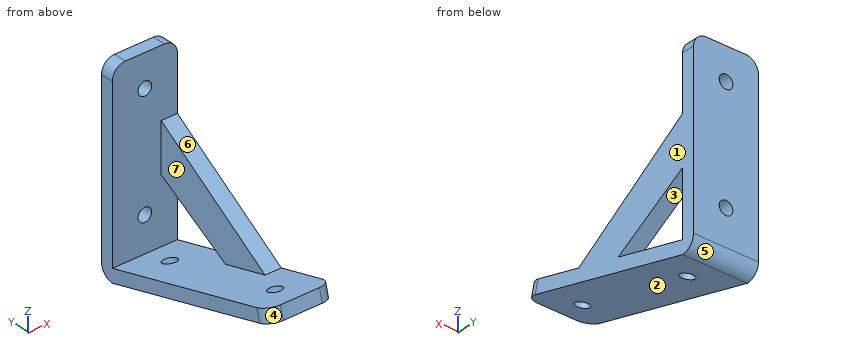
from build123d import *

# Parameters (mm, degrees)
SKETCH1_W           = 20
SKETCH1_H           = 60
BOSS_EXTRUDE1_DEPTH = 4
SKETCH6_W           = 20
SKETCH6_H           = 60
BOSS_EXTRUDE3_DEPTH = 4
FILLET6_R           = 4
SKETCH7_R           = 2.1
CUT_EXTRUDE3_DEPTH  = 4
SKETCH8_R           = 2.1
CUT_EXTRUDE4_DEPTH  = 4
FILLET7_R           = 4
FILLET8_R           = 4
FILLET9_R           = 4
FILLET10_R          = 4
BOSS_EXTRUDE5_DEPTH = 5


with BuildPart() as part:
    # Sketch1 → Boss-Extrude1 (new body)
    with BuildSketch(Plane(origin=(0, 0, 0), x_dir=(1, 0, 0), z_dir=(0, 1, 0))):
        Rectangle(SKETCH1_W, SKETCH1_H)
    extrude(amount=BOSS_EXTRUDE1_DEPTH)

    # Sketch6 → Boss-Extrude3 (add)
    with BuildSketch(Plane(origin=(0, -7.5, -27.990381057), x_dir=(-1, 0, 0), z_dir=(0, -0.25881904510251796, -0.9659258262890691))):
        with Locations((0, -22.235428647)):
            Rectangle(SKETCH6_W, SKETCH6_H)
    extrude(amount=-BOSS_EXTRUDE3_DEPTH)

    # Fillet6
    fillet6_edges = [part.edges().sort_by_distance(p)[0] for p in [
        (0, 4, -30),
    ]]
    fillet(fillet6_edges, radius=FILLET6_R - 0.0001)  # a hair under: the kernel refuses the full size

    # Sketch7 → Cut-Extrude3 (cut)
    with BuildSketch(Plane.XZ):
        with Locations(Location((0, 20, 0), (0, 0, 270))):
            Circle(SKETCH7_R)
        with Locations(Location((0, -15, 0), (0, 0, 270))):
            Circle(SKETCH7_R)
    extrude(amount=-CUT_EXTRUDE3_DEPTH, mode=Mode.SUBTRACT)

    # Sketch8 → Cut-Extrude4 (cut)
    with BuildSketch(Plane(origin=(0, -6.46472382, -24.126677752), x_dir=(1, 0, 0), z_dir=(0, 0.25881904510251796, 0.9659258262890691))):
        with Locations(Location((0, -2.771327032, 0), (0, 0, 270))):
            Circle(SKETCH8_R)
        with Locations(Location((0, -42.771327032, 0), (0, 0, 270))):
            Circle(SKETCH8_R)
    extrude(amount=-CUT_EXTRUDE4_DEPTH, mode=Mode.SUBTRACT)

    # Fillet7
    fillet7_edges = [part.edges().sort_by_distance(p)[0] for p in [
        (-10, -57.437911487, -12.539005641),
    ]]
    fillet(fillet7_edges, radius=FILLET7_R)

    # Fillet8
    fillet8_edges = [part.edges().sort_by_distance(p)[0] for p in [
        (10, -57.437911487, -12.539005641),
    ]]
    fillet(fillet8_edges, radius=FILLET8_R)

    # Fillet9
    fillet9_edges = [part.edges().sort_by_distance(p)[0] for p in [
        (10, 2, 30),
    ]]
    fillet(fillet9_edges, radius=FILLET9_R)

    # Fillet10
    fillet10_edges = [part.edges().sort_by_distance(p)[0] for p in [
        (-10, 2, 30),
    ]]
    fillet(fillet10_edges, radius=FILLET10_R)

    # Brace → Boss-Extrude5 (add)
    with BuildSketch(Plane(origin=(10, 0, 0), x_dir=(0, 0, -1), z_dir=(1, 0, 0))):
        Polygon((15.63686364, -38.149141432), (-9.141104722, 0), (5.858895278, 0), (19.519149316, -23.660254038), align=None)
    extrude(amount=-BOSS_EXTRUDE5_DEPTH)


solid = part.part
CAD build for the part. Positions are in the model's coordinates, mm. Face numbers are marked on the shaded views. A direction names the side the tool comes from. Round coordinates to 2 decimals unless told otherwise and drop trailing zeros. Order: outer loops, then holes, each group sorted by start corner. A loop starts at its lowest first (then second) coordinate and runs counter-clockwise, first axis right, second up. Notation, with made-up numbers: (76.25, 49.25) -> (134.25, 49.25) arc R21 cw to (134.25, 60.25) -> close; hole circle Ø4 at (4, -39). An arc over 180 degrees is marked (long way). Write item = value, one per line. Start each with the question number.
(1) Pin check, flat tips, straight feed: P1, Ø1.5, axis at x = -5, y = -16.5, coming from the +Z side; P2, Ø6, axis at x = -3.5, z = -7.5, coming from the -Y side; P3, Ø12, axis at x = 5.5, y = -32.5, coming from the -Z side; P4, Ø1, axis at y = -4.5, z = -24, coming from the -X side. Stop position of each tip, or through.
(2) Probe line 1 (X direction, y = 2.85, z = -15); line 2 (Y direction, x = -6.5, z = 24); line 3 (Z direction, x = 0.5, y = -19). List the from-to ranges inside material, lowest first. Write a range as [from, to].
(3) Cut at A-A, the plane z = 20. List the corners of the cut face in (x, y), then the cut area to 3 significant figures.
(4) Pull direction Z, two halves, no side cores. Call the marked faces 1, 2, 3 and 4: released by +Z, released by -Z, zero draft, split by the parting line, or undercut.
(5) Cut at C-C, the plane y = -2. List the corners of the cut face in (x, z), then the cut area to 3 significant figures.
(6) Which spindle directions (+Z, -Z, +X, -X, +Y, -Y) get a long thin tool onto all of the face, cutting with end or side? Do the marked faces 5, 6 and 7. Say none if no direction does.
Model answer:
q1.P1 = -21.24
q1.P2 = 0
q1.P3 = -22.9
q1.P4 = through
q2.line_1 = [-10, -2.1], [2.1, 10]
q2.line_2 = [0, 4]
q2.line_3 = [-24.91, -20.77]
q3.outline = (-10, 0) -> (-2.1, 0) -> (-2.1, 4) -> (-10, 4) -> close; (2.1, 0) -> (10, 0) -> (10, 4) -> (2.1, 4) -> close
q3.area = 63.2 mm2
q4.face_1 = zero draft
q4.face_2 = released by -Z
q4.face_3 = undercut
q4.face_4 = released by +Z
q5.outline = (-10, -29.46) -> (10, -29.46) -> (10, -25.32) -> (-10, -25.32) -> close; (5, -7.01) -> (10, -7.01) -> (10, 7.84) -> (5, 7.84) -> close
q5.area = 157 mm2
q6.face_5 = -Z, +X, -X, +Y
q6.face_6 = +Z, +X, -X
q6.face_7 = +Z, -X
